Could you check a few things on this model? Use its own coordinates, in mm. Coordinates: 2 decimals unless noted, no trailing zeros. Order: outer loops, then holes, each group sorted by start corner. A loop starts at its lowest first (then second) coordinate and runs counter-clockwise, first axis right, second up.
```python
from build123d import *

# Parameters (mm, degrees)
BOSS_EXTRUDE1_DEPTH = 1812.925
SKETCH2_R           = 10.31875
SKETCH2_R_2         = 7.14375
CUT_EXTRUDE1_DEPTH  = 51.8
SKETCH4_R           = 3.96875
CUT_EXTRUDE3_DEPTH  = 44.45
LPATTERN1_COUNT     = 15
LPATTERN1_PITCH     = 101.6


with BuildPart() as part:
    # Sketch1 → Boss-Extrude1 (new body)
    with BuildSketch(Plane.XY):
        Polygon((0, 0), (-50.8, 0), (-50.8, -3.175), (-3.175, -3.175), (-3.175, -50.8), (0, -50.8), align=None)
    extrude(amount=BOSS_EXTRUDE1_DEPTH)

    # Sketch2 → Cut-Extrude1 (cut, through all)
    with BuildSketch(Plane(origin=(0, 0, 0), x_dir=(1, 0, 0), z_dir=(0, 1, 0))):
        with Locations((-38.1, -37.30625)):
            Circle(SKETCH2_R)
        with Locations((-38.1, -1775.61875)):
            Circle(SKETCH2_R)
        with Locations((-33.3375, -93.6625)):
            Circle(SKETCH2_R_2)
        with Locations((-33.3375, -449.2625)):
            Circle(SKETCH2_R_2)
        with Locations((-33.3375, -855.6625)):
            Circle(SKETCH2_R_2)
        with Locations((-33.3375, -1262.0625)):
            Circle(SKETCH2_R_2)
        with Locations((-33.3375, -1719.2625)):
            Circle(SKETCH2_R_2)
    extrude(amount=-CUT_EXTRUDE1_DEPTH, mode=Mode.SUBTRACT)

    # Sketch4 → Cut-Extrude3 (cut)
    with BuildSketch(Plane(origin=(-2.029899632, 0, 893.163272881), x_dir=(1, 0, 0), z_dir=(0, 1, 0))):
        with Locations((-36.070100368, 697.900772881)):
            Circle(SKETCH4_R)
    cut_extrude3 = extrude(amount=-CUT_EXTRUDE3_DEPTH, mode=Mode.SUBTRACT)

    # LPattern1: Cut-Extrude3 ×15
    with Locations(*[(0, 0, i * LPATTERN1_PITCH) for i in range(1, LPATTERN1_COUNT)]):
        add(cut_extrude3, mode=Mode.SUBTRACT)


solid = part.part
```
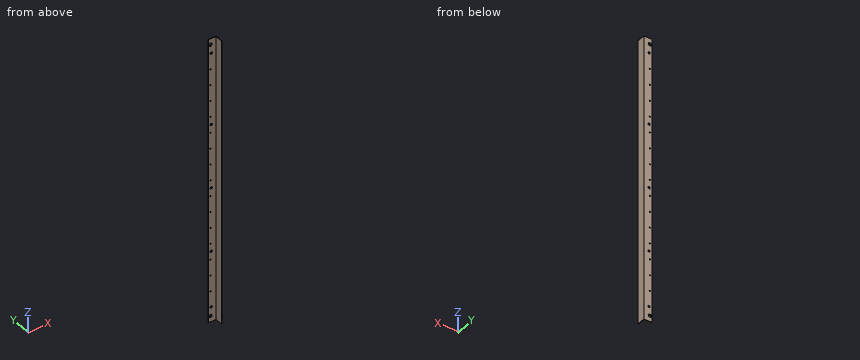
Item 1: For pin 1 Ø10.5 at (x, z) = (-38.1, 804.86) entering from +Y; pin 2 Ø18.5 at (x, z) = (-33.34, 855.66) entering from -Y (3 decimals); pin 3 Ø6.5 at (x, z) = (-38.1, 1617.66) entering from +Y; pin 4 Ø8 at (y, z) = (-28.5, 1508) entering from -X (3 decimals), each with a flat end and sliding along its axis, tell me the tip position at first contact or that it passes through.
Item 2: Suppose I cut it at A-A (z = 550). List the corners of the cut face in (x, y) for me (3 decimals), and give its area (4 significant figures).
Item 3: Suppose I cut it at B-B (y = -30). List the corners of the cut face in (x, z) for me (3 decimals).
Item 4: I need wall thicknesses on line 1 (X direction, y = -12, z = 93.5) (3 decimals). Which ranges of the line are inside material? Lowest first, please.
Geometry results:
1. pin 1: stops at y = 0
1. pin 2: stops at y = -3.175
1. pin 3: passes through
1. pin 4: stops at x = -3.175
2. outline: (-50.8, -3.175) - (-3.175, -3.175) - (-3.175, -50.8) - (0, -50.8) - (0, 0) - (-50.8, 0) - close
2. area: 312.5 mm2
3. outline: (-3.175, 0) - (0, 0) - (0, 1812.925) - (-3.175, 1812.925) - close
4. line 1: x = -3.175 to 0
